The model under review builds one solid part; all positions refer to its coordinate system, in mm. A direction names the side the tool comes from. Round coordinates to 2 decimals unless told otherwise and drop trailing zeros. Write each loop counter-clockwise with the first axis right and the second up, starting at its lowest first coordinate (ties: lowest second). Pieces come first, ordered by that corner, then holes. Notation, with made-up numbers: (85, -11.5) - (103, -11.5) arc R13 cw to (103, 1.5) - close; hole circle Ø6 at (18, 81). An arc over 180 degrees is marked (long way). Return JSON: item names as keys, results as strings.
from build123d import *

# Parameters (mm, degrees)
SKETCH_1_R          = 10.5
EXTRUDE_1_DEPTH     = 45
EXTRUDE_2_DEPTH     = 10
SKETCH_3_R          = 6.25
EXTRUDE_3_DEPTH     = 10
FILLET_1_R          = 0.5
SKETCH_4_R          = 3.905073707
CUT_EXTRUDE_1_DEPTH = 60


with BuildPart() as part:
    # 草图1 → 凸台-拉伸1 (new body)
    with BuildSketch(Plane.XY):
        with Locations(Location((0, 0, 0), (0, 0, 180))):
            Circle(SKETCH_1_R)
    extrude(amount=EXTRUDE_1_DEPTH)

    # 草图2 → 凸台-拉伸2 (add)
    with BuildSketch(Plane(origin=(0, 0, 0), x_dir=(-1, 0, 0), z_dir=(0, 0, -1))):
        Polygon((6.805240256, -7.996168149), (10.327504878, 1.895426866), (3.522264622, 9.891595015), (-6.805240256, 7.996168149), (-10.327504878, -1.895426866), (-3.522264622, -9.891595015), align=None)
    extrude(amount=EXTRUDE_2_DEPTH)

    # 草图3 → 凸台-拉伸3 (add)
    with BuildSketch(Plane(origin=(0, 0, -10), x_dir=(-1, 0, 0), z_dir=(0, 0, -1))):
        Circle(SKETCH_3_R)
    extrude(amount=EXTRUDE_3_DEPTH)

    # 圆角1
    fillet_1_edges = [part.edges().sort_by_distance(p)[0] for p in [
        (6.25, 0, -20),
        (10.5, 0, 45),
    ]]
    fillet(fillet_1_edges, radius=FILLET_1_R)

    # 草图4 → 切除-拉伸1 (cut)
    with BuildSketch(Plane(origin=(0, 0, -20), x_dir=(-1, 0, 0), z_dir=(0, 0, -1))):
        Circle(SKETCH_4_R)
    extrude(amount=-CUT_EXTRUDE_1_DEPTH, mode=Mode.SUBTRACT)


solid = part.part
(1) Add section A-A (y = 0). Write out the cut boundary in (x, z).
Filled in:
{"outline": "(-10.5, 0) - (-9.65, 0) - (-9.65, -10) - (-6.25, -10) - (-6.25, -19.5) arc R0.5 ccw to (-5.75, -20) - (-3.91, -20) - (-3.91, 40) - (3.91, 40) - (3.91, -20) - (5.75, -20) arc R0.5 ccw to (6.25, -19.5) - (6.25, -10) - (9.65, -10) - (9.65, 0) - (10.5, 0) - (10.5, 44.5) arc R0.5 ccw to (10, 45) - (-10, 45) arc R0.5 ccw to (-10.5, 44.5) - close"}
(2) For faces 1 (the flat face through (-6.97, 5.84, -4.93)), 2 (the flat face through (-2, -10, 0)), 3 (the flat face through (5, -4, -10)), 4 (the flat face through (7.4, -6.2, 0)), list the 3-axis set-ups (+Z, -Z, +X, -X, +Y, -Y) from which the entire face can be reached by the end or side of a thin tool; tool diameter is ignored.
Filled in:
{"face 1": "-Z, -X, +Y", "face 2": "-Z, -X, -Y", "face 3": "-Z", "face 4": "-Z, +X, -Y"}
(3) Wall thickness on line 1 (Y direction, x = 0, z = 5.5); line 2 (Z direction, x = 2, y = -6.75); line 3 (Y direction, x = -2, z = 12.5): over which ranges is each line inside the solid? List them lowest first.
Filled in:
{"line 1": "y = -10.5 to -3.91, 3.91 to 10.5", "line 2": "z = -10 to 45", "line 3": "y = -10.31 to -3.35, 3.35 to 10.31"}
(4) Add section B-B (z = -15). Write out the cut boundary in (x, y).
Filled in:
{"outline": "circle Ø12.5 at (0, 0); hole circle Ø7.81 at (0, 0)"}
(5) Add section D-D (z = 11.5). Write out the cut boundary in (x, y).
Filled in:
{"outline": "circle Ø21 at (0, 0); hole circle Ø7.81 at (0, 0)"}
(6) Add section C-C (x = 0). Write out the cut boundary in (y, z).
Filled in:
{"outline": "(-10.5, 0) - (-9.25, 0) - (-9.25, -10) - (-6.25, -10) - (-6.25, -19.5) arc R0.5 ccw to (-5.75, -20) - (-3.91, -20) - (-3.91, 40) - (3.91, 40) - (3.91, -20) - (5.75, -20) arc R0.5 ccw to (6.25, -19.5) - (6.25, -10) - (9.25, -10) - (9.25, 0) - (10.5, 0) - (10.5, 44.5) arc R0.5 ccw to (10, 45) - (-10, 45) arc R0.5 ccw to (-10.5, 44.5) - close"}
(7) Clearance check with flat-ended pins moving along their axes: pin 1 Ø2 at (x, z) = (6.5, -3) entering from +Y; pin 2 Ø1 at (y, z) = (4.5, 24) entering from -X; pin 3 Ø1 at (x, z) = (5.5, -5.5) entering from +Y. State where each tip first meets the part, or that it passes through.
Filled in:
{"pin 1": "stops at y = 8.24", "pin 2": "stops at x = -9.71", "pin 3": "stops at y = 8.33"}
